from build123d import *

# Parameters (mm, degrees)
SKETCH1_R           = 6
SKETCH1_R_2         = 3.75
SKETCH1_R_3         = 1
BOSS_EXTRUDE1_DEPTH = 5


with BuildPart() as part:
    # Sketch1 → Boss-Extrude1 (new body)
    with BuildSketch(Plane(origin=(0, 0, 0), x_dir=(1, 0, 0), z_dir=(0, 1, 0))):
        with BuildLine():
            Line((65.5, 12.5), (62, 12.5))
            Line((62, 12.5), (62, 0))
            Line((62, 0), (0, 0))
            Line((0, 0), (0, 48))
            Line((0, 48), (62, 48))
            Line((62, 48), (62, 35.5))
            Line((62, 35.5), (65.5, 35.5))
            ThreePointArc((65.5, 35.5), (68, 33), (65.5, 30.5))
            Line((65.5, 30.5), (62, 30.5))
            Line((62, 30.5), (62, 26.5))
            Line((62, 26.5), (65.5, 26.5))
            ThreePointArc((65.5, 26.5), (68, 24), (65.5, 21.5))
            Line((65.5, 21.5), (62, 21.5))
            Line((62, 21.5), (62, 17.5))
            Line((62, 17.5), (65.5, 17.5))
            ThreePointArc((65.5, 17.5), (68, 15), (65.5, 12.5))
        make_face()
        with Locations(Location((10, 10, 0), (0, 0, 270))):
            Circle(SKETCH1_R, mode=Mode.SUBTRACT)
        with Locations(Location((10, 38, 0), (0, 0, 270))):
            Circle(SKETCH1_R, mode=Mode.SUBTRACT)
        with Locations(Location((25, 24, 0), (0, 0, 270))):
            Circle(SKETCH1_R_2, mode=Mode.SUBTRACT)
        with Locations(Location((65.5, 15, 0), (0, 0, 270))):
            Circle(SKETCH1_R_3, mode=Mode.SUBTRACT)
        with Locations(Location((65.5, 24, 0), (0, 0, 270))):
            Circle(SKETCH1_R_3, mode=Mode.SUBTRACT)
        with Locations(Location((65.5, 33, 0), (0, 0, 270))):
            Circle(SKETCH1_R_3, mode=Mode.SUBTRACT)
    extrude(amount=BOSS_EXTRUDE1_DEPTH)


solid = part.part
Source: CAD feature listing. Evaluate the final solid. Frame: model axes, mm. A direction names the side the tool comes from. Coordinates: 2 decimals unless noted, no trailing zeros. Loops run counter-clockwise (first coordinate to the right, second up) from the corner with the lowest first, then second, coordinate; pieces in that order, holes last. Notation, with made-up numbers: M 59.5,3.5 L 114.5,3.5 A17 cw 114.5,30.5 Z; hole C 3,-15 d10. An arc over 180 degrees is marked long. Answer in a Markdown table with one row per item.
Q1. Draft query along X for faces 1 (the cylindrical face through (6.35, 2.46, -42.76)), 2 (the flat face through (64, 2, -35.5)), 3 (the cylindrical face through (64.61, 2.46, -32.54)), 4 (the flat face through (62, 2, -6)). Return one class per face: pulls with the +X half, pulls with the -X half, needs draft (parallel to the pull), parting line crosses it, or undercut.
Answers below:
| item | result |
|---|---|
| face 1 | undercut |
| face 2 | needs draft |
| face 3 | undercut |
| face 4 | pulls with the +X half |
Q2. Ray query, probe 1 along Z at (x, y) = (65.5, 3.3); probe 2 along X at (y, z) = (4.05, -24); probe 3 along Z at (x, y) = (63, 2.85). Return the intervals inside material, ascending. Write a range as from..to.
Answers below:
| item | result |
|---|---|
| probe 1 | z = -35.5..-34, -32..-30.5, -26.5..-25, -23..-21.5, -17.5..-16, -14..-12.5 |
| probe 2 | x = 0..21.25, 28.75..64.5, 66.5..68 |
| probe 3 | z = -35.5..-30.5, -26.5..-21.5, -17.5..-12.5 |
Q3. Section C-C on z = -24. Return the cut outline in (x, y), plus the area to 4 significant figures.
Answers below:
| item | result |
|---|---|
| outline | M 0,0 L 21.25,0 L 21.25,5 L 0,5 Z; M 28.75,0 L 64.5,0 L 64.5,5 L 28.75,5 Z; M 66.5,0 L 68,0 L 68,5 L 66.5,5 Z |
| area | 292.5 mm^2 |
Q4. Section D-D on y = 2.35. Return the cut outline in (x, z).
Answers below:
| item | result |
|---|---|
| outline | M 0,-48 L 62,-48 L 62,-35.5 L 65.5,-35.5 A2.5 ccw 65.5,-30.5 L 62,-30.5 L 62,-26.5 L 65.5,-26.5 A2.5 ccw 65.5,-21.5 L 62,-21.5 L 62,-17.5 L 65.5,-17.5 A2.5 ccw 65.5,-12.5 L 62,-12.5 L 62,0 L 0,0 Z; hole C 10,-38 d12; hole C 10,-10 d12; hole C 25,-24 d7.5; hole C 65.5,-33 d2; hole C 65.5,-24 d2; hole C 65.5,-15 d2 |
Q5. Set-up query: faces 5 (the flat face through (64, 2, -17.5)), 6 (the flat face through (62, 2, -42)), 7 (the flat face through (64, 2, -12.5)). Return all of +Z, -Z, +X, -X, +Y, -Y with unobstructed straight access to the full face (end or side cutting, diameter ignored); none if empty.
Answers below:
| item | result |
|---|---|
| face 5 | +X, +Y, -Y |
| face 6 | -Z, +X, +Y, -Y |
| face 7 | +Z, +X, +Y, -Y |
Q6. Section A-A on x = 25. Return the cut outline in (y, z).
Answers below:
| item | result |
|---|---|
| outline | M 0,-48 L 5,-48 L 5,-27.75 L 0,-27.75 Z; M 0,-20.25 L 5,-20.25 L 5,0 L 0,0 Z |
Q7. First-contact query: pin 1 (2 mm diameter, centred on y = 3, z = -19, fed in from +X); pin 2 (3 mm diameter, centred on x = 64, y = 2.5, fed in from +Z); pin 3 (3 mm diameter, centred on x = 64, y = 3.5, fed in from -Z). Flat tips, straight axial feed; report the tip coordinate or a pass-through.
Answers below:
| item | result |
|---|---|
| pin 1 | stops at x = 62 |
| pin 2 | stops at z = -12.5 |
| pin 3 | stops at z = -35.5 |
Q8. Section B-B on z = -10. Return the cut outline in (x, y), plus the area to 3 significant figures.
Answers below:
| item | result |
|---|---|
| outline | M 0,0 L 4,0 L 4,5 L 0,5 Z; M 16,0 L 62,0 L 62,5 L 16,5 Z |
| area | 250 mm^2 |
